Source: CAD feature listing. Evaluate the final solid. Frame: model axes, mm. Coordinates: 2 decimals unless noted, no trailing zeros. Order: outer loops, then holes, each group sorted by start corner. A loop starts at its lowest first (then second) coordinate and runs counter-clockwise, first axis right, second up. Notation, with made-up numbers: (34, 6.5) -> (42, 6.5) arc R15 ccw to (42, 35.5) -> close; hole circle Ø11 at (73.25, 46.5). An arc over 180 degrees is marked (long way). Write item = value, one per line. Start each with the question number.
Item 1: Contact query for flat-ended pins moving along their axis: pin 1 (2 mm diameter, centred on x = 46, y = 20.5, fed in from +Z); pin 2 (12 mm diameter, centred on y = 0.5, z = -70, fed in from -X); pin 3 (5 mm diameter, centred on x = 44.5, y = 15.5, fed in from +Z). Output: stop coordinate, or through.
Item 2: Ray query, line 1 along X through (y, z) = (12, -267); line 2 along X through (y, z) = (-0.5, -283); line 3 along Z through (x, y) = (43.5, 9.5). Return the intervals inside material, ascending. Write a range as [from, to].
Item 3: Section query A-A (z = -306). Output: boundary loops of the cut face in (x, y).
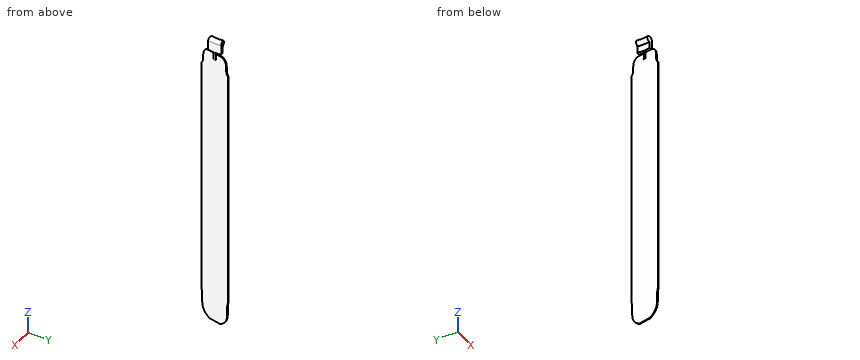
```python
from build123d import *

# Parameters (mm, degrees)
REVOLVE_1_ANGLE          = 20
EXTRUDE_1_DEPTH          = 10
EXTRUDE_2_DEPTH          = 360
EXTRUDE_2_DEPTH_BACK     = 8
CUT_EXTRUDE_1_DEPTH      = 354.460525949
CUT_EXTRUDE_1_DEPTH_BACK = 354.460525949
CUT_EXTRUDE_2_DEPTH      = 354.460526061
CUT_EXTRUDE_2_DEPTH_BACK = 354.460526061


# Read off the part's stored shape, not the designer's step: 旋转1
with BuildPart() as part:
    # 旋转1 outline → 旋转1 (revolve)
    with BuildSketch(Plane(origin=(-4.145534285, 10.115302746, 0), x_dir=(0.9848077530122078, -0.17364817766693175, 0), z_dir=(-0.17364817766693175, -0.9848077530122078, 0))):
        with BuildLine():
            Line((48.69007377, 18.497782452), (48.69007377, 30.884801913))
            ThreePointArc((48.69007377, 30.884801913), (42.390721279, 33.49407915), (44.999998514, 27.194726658))
            Line((44.999998514, 27.194726658), (44.999998514, 18.497782452))
            Line((44.999998514, 18.497782452), (48.69007377, 18.497782452))
        make_face()
    revolve(axis=Axis((-4.145534285, 10.115302746, 0), (0, 0, 1)), revolution_arc=REVOLVE_1_ANGLE)

    # 草图2 → 凸台-拉伸1 (add)
    with BuildSketch(Plane(origin=(0, 0, 18.497782452), x_dir=(-1, 0, 0), z_dir=(0, 0, -1))):
        with BuildLine():
            Line((-43.804827858, 10.115302746), (-43.804827858, 8.790890094))
            ThreePointArc((-43.804827858, 8.790890094), (-42.230547682, 8.757264374), (-41.433540442, 10.115302746))
            Line((-41.433540442, 10.115302746), (-43.804827858, 10.115302746))
        make_face()
        with BuildLine():
            Line((-43.804827858, 11.439715397), (-43.804827858, 10.115302746))
            Line((-43.804827858, 10.115302746), (-41.433540442, 10.115302746))
            ThreePointArc((-41.433540442, 10.115302746), (-42.230547682, 11.473341118), (-43.804827858, 11.439715397))
        make_face()
        with BuildLine():
            ThreePointArc((-43.804827858, 11.439715397), (-44.544539485, 10.115302746), (-43.804827858, 8.790890094))
            Line((-43.804827858, 8.790890094), (-43.804827858, 10.115302746))
            Line((-43.804827858, 10.115302746), (-43.804827858, 11.439715397))
        make_face()
    extrude(amount=EXTRUDE_1_DEPTH)

    # 草图3 → 凸台-拉伸2 (add, two sides: drawn at the far end of the back side and taken through both)
    with BuildSketch(Plane(origin=(0, 0, 8.497782452), x_dir=(-1, 0, 0), z_dir=(0, 0, -1)).offset(-EXTRUDE_2_DEPTH_BACK)):
        Polygon((-45.891658823, 29.456257554), (-46.915436985, 29.275737842), (-40.047450695, -9.674547938), (-39.023672534, -9.494028226), align=None)
    extrude(amount=EXTRUDE_2_DEPTH + EXTRUDE_2_DEPTH_BACK)

    # 草图4 → 切除-拉伸1 (cut, two sides: drawn at the far end of the back side and taken through both)
    with BuildSketch(Plane(origin=(40.494317434, -7.140240729, 0), x_dir=(0, 0, -1), z_dir=(0.9848077530122087, -0.17364817766692764, 0)).offset(-CUT_EXTRUDE_1_DEPTH_BACK)):
        with BuildLine():
            Line((-16.497782452, 36.977753739), (-16.497782452, 27.931634297))
            add(Edge.make_bspline(
                [(-16.497782452, 27.931634297), (-15.119446691, 32.122246332), (-9.533617097, 34.35083792), (-2.34707738, 33.953128128), (2.582817502, 34.306427345), (5.20587008, 36.009348447), (6.100812574, 36.977753739)],
                knots=[0, 0, 0, 0, 0.299327733, 0.443712894, 0.582270155, 0.686413385, 0.686413385, 0.686413385, 0.686413385], degree=3))
            Line((6.100812574, 36.977753739), (-16.497782452, 36.977753739))
        make_face()
        with BuildLine():
            Line((-16.497782452, 6.472716459), (-16.497782452, -2.573402982))
            Line((-16.497782452, -2.573402982), (6.100812574, -2.573402982))
            add(Edge.make_bspline(
                [(-16.497782452, 6.472716459), (-15.119446691, 2.282104425), (-9.533617097, 0.053512837), (-2.34707738, 0.451222629), (2.582817502, 0.097923412), (5.20587008, -1.604997691), (6.100812574, -2.573402982)],
                knots=[0, 0, 0, 0, 0.299327733, 0.443712894, 0.582270155, 0.686413385, 0.686413385, 0.686413385, 0.686413385], degree=3))
        make_face()
    extrude(amount=CUT_EXTRUDE_1_DEPTH + CUT_EXTRUDE_1_DEPTH_BACK, mode=Mode.SUBTRACT)

    # 草图5 → 切除-拉伸2 (cut, two sides: drawn at the far end of the back side and taken through both)
    with BuildSketch(Plane(origin=(40.494317434, -7.140240729, 0), x_dir=(0, 0, -1), z_dir=(0.9848077530122087, -0.17364817766692764, 0)).offset(-CUT_EXTRUDE_2_DEPTH_BACK)):
        with BuildLine():
            Line((351.502217548, 36.977753739), (316.754779292, 36.977753739))
            add(Edge.make_bspline(
                [(351.502217548, 25.127512161), (347.967875432, 31.121714431), (339.410781642, 38.011527911), (319.00267796, 34.531851346), (316.754779292, 36.977753739)],
                knots=[0, 0, 0, 0, 0.348264384, 0.764472807, 0.764472807, 0.764472807, 0.764472807], degree=3))
            Line((351.502217548, 25.127512161), (351.502217548, 36.977753739))
        make_face()
        with BuildLine():
            Line((351.502217548, -2.573402982), (351.502217548, 9.276838596))
            add(Edge.make_bspline(
                [(351.502217548, 9.276838596), (347.967875432, 3.282636325), (339.410781642, -3.607177155), (319.00267796, -0.127500589), (316.754779292, -2.573402982)],
                knots=[0, 0, 0, 0, 0.348264384, 0.764472807, 0.764472807, 0.764472807, 0.764472807], degree=3))
            Line((316.754779292, -2.573402982), (351.502217548, -2.573402982))
        make_face()
    extrude(amount=CUT_EXTRUDE_2_DEPTH + CUT_EXTRUDE_2_DEPTH_BACK, mode=Mode.SUBTRACT)


solid = part.part
```
Computed:
q1.pin_1 = 16.5
q1.pin_2 = 39.73
q1.pin_3 = 34.28
q2.line_1 = [42.81, 43.87]
q2.line_2 = [40.61, 41.67]
q2.line_3 = [8.5, 33.45]
q3.outline = (39.02, -9.49) -> (40.05, -9.67) -> (46.92, 29.28) -> (45.89, 29.46) -> close
